Can you work these out from the model? Positions are in its coordinate system, mm. A direction names the side the tool comes from. Coordinates: 2 decimals unless noted, no trailing zeros. Order: outer loops, then holes, each group sorted by start corner. A loop starts at its lowest first (then second) coordinate and runs counter-clockwise, first axis right, second up. Notation, with made-up numbers: (72, 32) -> (91, 32) arc R25 cw to (91, 58) -> close; hole circle Ø8 at (55.25, -1.5). An arc over 180 degrees is marked (long way). Answer as a JSON object with one key per item and string values. Group by question number.
(1) I want a section at D-D, the plane z = -11. List the corners of the cut face in (x, y) for me, plus the area to 3 significant figures.
(2) I want a section at B-B, the plane z = -32.5. List the corners of the cut face in (x, y) for me.
(3) For pin 1 (4 mm diameter, centred on x = 53.5, y = 15, fed in from +Z); pin 2 (1.8 mm diameter, centred on y = 23, z = -18.64, fed in from -X); pin 3 (1.5 mm diameter, centred on x = 35, y = 15, fed in from +Z), each with a flat end and sliding along its axis, tell me the tip position at first contact or that it passes through.
(4) I want a section at C-C, the plane y = 7. List the corners of the cut face in (x, z) for me, plus the area to 3 significant figures.
(5) Which directions (+Z, -Z, +X, -X, +Y, -Y) give clear straight access to the entire face, cutting with the end or side of a thin tool? Please do faces 1 (the flat face through (37, 17, -75)), 2 (the flat face through (8, 2, 5)), 3 (the cylindrical face through (26.443, 13.093, 4.93)), 4 (the flat face through (13, 2, -12.5)).
(6) If we mould it in two halves opening along Y, with no side actions, what happens to faces 5 (the flat face through (57, 2, 5)), 6 (the cylindrical face through (2.958, 22.934, -17.145)), 7 (the cylindrical face through (26.443, 16.907, -70.07)), 8 (the flat face through (13, 4, -10))? For each: pulls with the +Y half, pulls with the -Y half, needs draft (parallel to the pull), parting line crosses it, or undercut.
(7) I want a section at A-A, the plane x = 32.5. State how many separate pieces and enclosed holes the cut face has, plus the area to 3 significant figures.
(8) I need wall thicknesses on line 1 (Z direction, x = 14.5, y = 28.5); line 2 (X direction, y = 23, z = -6.5); line 3 (Y direction, x = 32.5, z = 5) (3 decimals). Which ranges of each line are inside material? Lowest first, please.
from build123d import *

# Parameters (mm, degrees)
SKETCH1_W           = 65
SKETCH1_H           = 65
SKETCH1_W_2         = 53
SKETCH1_H_2         = 53
BOSS_EXTRUDE1_DEPTH = 30
SKETCH3_R           = 11.5125
CUT_EXTRUDE2_DEPTH  = 97.695398029
SKETCH2_R           = 4.4625
BOSS_EXTRUDE2_DEPTH = 17.5
BOSS_EXTRUDE3_START = -82.5
SKETCH2_2_R         = 4.4625
BOSS_EXTRUDE3_DEPTH = 17.5
CUT_EXTRUDE3_REACH  = 124.984
SKETCH5_R           = 6.35
SKETCH5_R_2         = 4.4625
BOSS_EXTRUDE4_DEPTH = 10
BOSS_EXTRUDE5_START = 10
SKETCH6_R           = 6.35
SKETCH6_R_2         = 4.4625
BOSS_EXTRUDE5_DEPTH = 10
SKETCH7_R           = 1.5
CUT_EXTRUDE4_DEPTH  = 10
BOSS_EXTRUDE6_START = 30
BOSS_EXTRUDE6_DEPTH = 4
BOSS_EXTRUDE8_DEPTH = 4
FILLET3_R           = 1


with BuildPart() as part:
    # Sketch1 → Boss-Extrude1 (new body)
    with BuildSketch(Plane(origin=(0, 0, 0), x_dir=(1, 0, 0), z_dir=(0, 1, 0))):
        with Locations((32.5, 32.5)):
            Rectangle(SKETCH1_W, SKETCH1_H)
        with Locations((32.5, 32.5)):
            Rectangle(SKETCH1_W_2, SKETCH1_H_2, mode=Mode.SUBTRACT)
    extrude(amount=BOSS_EXTRUDE1_DEPTH)

    # Sketch3 → Cut-Extrude2 (cut, through all)
    with BuildSketch(Plane(origin=(65, 0, 0), x_dir=(0, 0, -1), z_dir=(1, 0, 0))):
        with Locations((32.5, 15)):
            Circle(SKETCH3_R)
    extrude(amount=-CUT_EXTRUDE2_DEPTH, mode=Mode.SUBTRACT)

    # Sketch2 → Boss-Extrude2 (add)
    with BuildSketch(Plane.XY):
        with Locations(Location((32.5, 15, 0), (0, 0, 180))):
            Circle(SKETCH2_R)
    extrude(amount=BOSS_EXTRUDE2_DEPTH)

    # Sketch2<2> → Boss-Extrude3 (add)
    with BuildSketch(Plane.XY.offset(BOSS_EXTRUDE3_START)):
        with Locations(Location((32.5, 15, 0), (0, 0, 180))):
            Circle(SKETCH2_2_R)
    extrude(amount=BOSS_EXTRUDE3_DEPTH)

    # Sketch4 → Cut-Extrude3 (cut, up to next)
    with BuildSketch(Plane.XY.offset(17.5), mode=Mode.PRIVATE) as cut_extrude3_sk1:
        with BuildLine():
            Line((30.185, 17.455890877), (34.815, 17.455890877))
            ThreePointArc((34.815, 17.455890877), (32.5, 11.625), (30.185, 17.455890877))
        make_face()
    cut_extrude3_tool1 = extrude(cut_extrude3_sk1.sketch, amount=-CUT_EXTRUDE3_REACH, mode=Mode.PRIVATE) & part.part
    add(cut_extrude3_tool1.solids().sort_by_distance((32.5, 14.748295, 17.5))[0], mode=Mode.SUBTRACT)

    # Sketch5 → Boss-Extrude4 (add)
    with BuildSketch(Plane.XY):
        with Locations(Location((32.5, 15, 0), (0, 0, 180))):
            Circle(SKETCH5_R)
        with Locations((32.5, 15)):
            Circle(SKETCH5_R_2, mode=Mode.SUBTRACT)
    extrude(amount=BOSS_EXTRUDE4_DEPTH)

    # Sketch6 → Boss-Extrude5 (add)
    with BuildSketch(Plane(origin=(0, 0, -65), x_dir=(-1, 0, 0), z_dir=(0, 0, -1)).offset(BOSS_EXTRUDE5_START)):
        with Locations((-32.5, 15)):
            Circle(SKETCH6_R)
        with Locations(Location((-32.5, 15, 0), (0, 0, 180))):
            Circle(SKETCH6_R_2, mode=Mode.SUBTRACT)
    extrude(amount=-BOSS_EXTRUDE5_DEPTH)

    # Sketch7 → Cut-Extrude4 (cut)
    with BuildSketch(Plane.ZY):
        with Locations((-46.356406461, 23)):
            Circle(SKETCH7_R)
        with Locations(Location((-46.356406461, 7, 0), (0, 0, 180))):
            Circle(SKETCH7_R)
        with Locations(Location((-18.643593539, 23, 0), (0, 0, 180))):
            Circle(SKETCH7_R)
        with Locations((-18.643593539, 7)):
            Circle(SKETCH7_R)
    extrude(amount=-CUT_EXTRUDE4_DEPTH, mode=Mode.SUBTRACT)

    # Sketch8 → Boss-Extrude6 (add)
    with BuildSketch(Plane(origin=(30, 30, 0), x_dir=(0, 0, 1), z_dir=(0, -1, 0)).offset(BOSS_EXTRUDE6_START)):
        Polygon((0, -35), (6.5, -35), (6.5, -31), (6.5, -27), (2.5, -27), (2.5, -31), (0, -31), align=None)
    boss_extrude6 = extrude(amount=-BOSS_EXTRUDE6_DEPTH)

    # Sketch9 → Boss-Extrude8 (add)
    with BuildSketch(Plane.XZ):
        Polygon((17, -59), (17, -52.5), (13, -52.5), (9, -52.5), (9, -56.5), (13, -56.5), (13, -59), align=None)
    boss_extrude8 = extrude(amount=-BOSS_EXTRUDE8_DEPTH)

    # Mirror1: Boss-Extrude6 across plane
    add(boss_extrude6.mirror(Plane.ZY.offset(-32.5)))

    # Mirror2: Boss-Extrude8 across plane
    add(boss_extrude8.mirror(Plane.XY.offset(-32.5)))

    # Fillet3
    fillet3_edges = [part.edges().sort_by_distance(p)[0] for p in [
        (61, 2, 2.5),
        (61, 2, 0),
        (17, 2, -59),
        (13, 2, -59),
        (13, 2, -56.5),
        (4, 2, 2.5),
        (4, 2, 0),
        (13, 2, -6),
        (17, 2, -6),
        (13, 2, -8.5),
    ]]
    fillet(fillet3_edges, radius=FILLET3_R)


solid = part.part
Computed values:
{
 "1": {"outline": "(0, 0) -> (6, 0) -> (6, 30) -> (0, 30) -> close; (9, 0) -> (17, 0) -> (17, 4) -> (9, 4) -> close; (59, 0) -> (65, 0) -> (65, 30) -> (59, 30) -> close", "area": "392 mm2"},
 "2": {"outline": "(0, 0) -> (6, 0) -> (6, 3.49) -> (0, 3.49) -> close; (0, 26.51) -> (6, 26.51) -> (6, 30) -> (0, 30) -> close; (59, 0) -> (65, 0) -> (65, 3.49) -> (59, 3.49) -> close; (59, 26.51) -> (65, 26.51) -> (65, 30) -> (59, 30) -> close"},
 "3": {"pin 1": "stops at z = 0", "pin 2": "stops at x = 59", "pin 3": "stops at z = -59"},
 "4": {"outline": "(0, -65) -> (65, -65) -> (65, -40.78) -> (59, -40.78) -> (59, -59) -> (6, -59) -> (6, -47.86) -> (0, -47.86) -> close; (0, -44.86) -> (6, -44.86) -> (6, -40.78) -> (0, -40.78) -> close; (0, -24.22) -> (6, -24.22) -> (6, -20.14) -> (0, -20.14) -> close; (0, -17.14) -> (6, -17.14) -> (6, -6) -> (59, -6) -> (59, -24.22) -> (65, -24.22) -> (65, 0) -> (0, 0) -> close", "area": "1,180 mm2"},
 "5": {"face 1": "-Z", "face 2": "+Z, +Y, -Y", "face 3": "+Z", "face 4": "+Y, -Y"},
 "6": {"face 5": "needs draft", "face 6": "undercut", "face 7": "parting line crosses it", "face 8": "pulls with the +Y half"},
 "7": {"separate pieces": "3", "enclosed holes": "0", "area": "611 mm2"},
 "8": {"line 1": "z = -65 to -59, -6 to 0", "line 2": "x = 0 to 6, 59 to 65", "line 3": "y = 8.65 to 11.625, 17.456 to 21.35"}
}
